Verification items for this drawing (mm, ordinates from the low corner). Coordinates: 2 decimals unless noted, no trailing zeros. Order: outer loops, then holes, each group sorted by start corner. A loop starts at its lowest first (then second) coordinate and runs counter-clockwise, first axis right, second up. Notation, with made-up numbers: M 36.5,-5.5 L 82.5,-5.5 A17 cw 82.5,19.5 Z; hole C 46,3 d11. An arc over 180 degrees is marked long. Use CSV: the item, a comma, the result in double quotes. Start each with the question number.
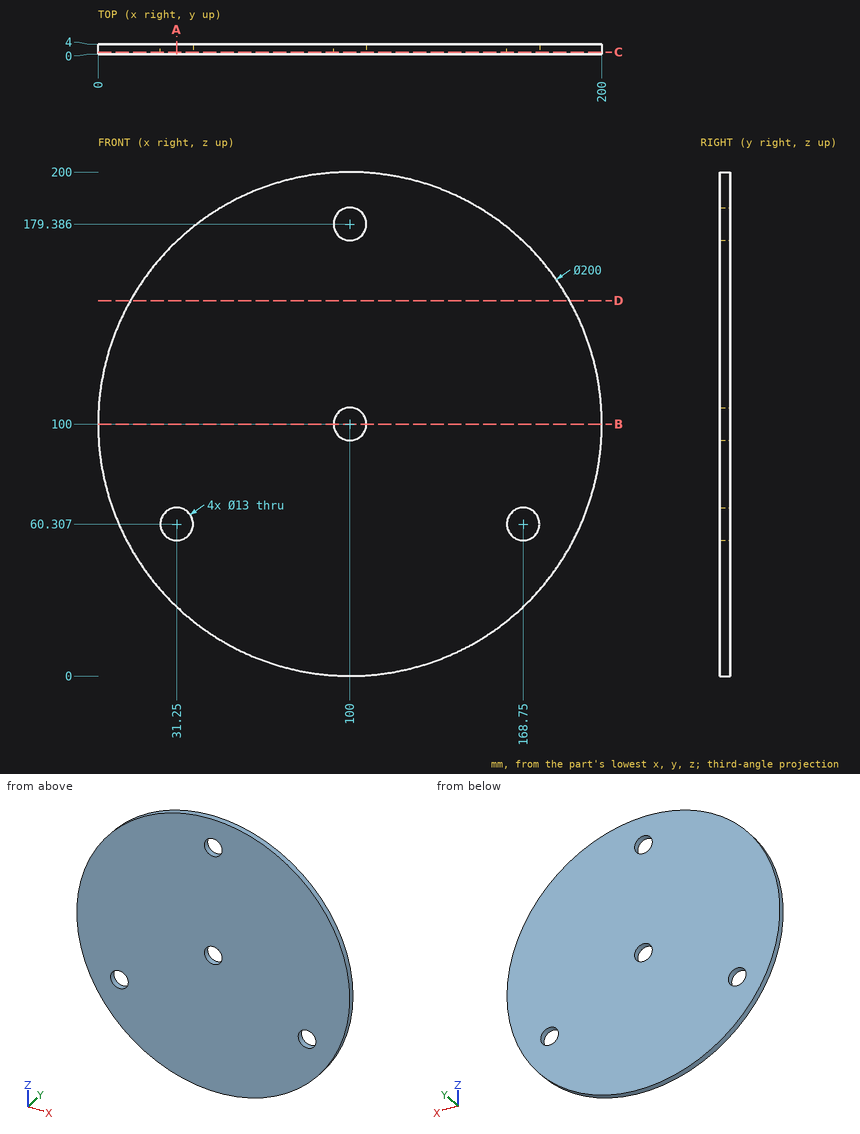
1) Section check B-B on z = 100. Record the boundary of the cut face in (x, y), then the cut area to 3 significant figures.
2) Section check D-D on z = 149. Record the boundary of the cut face in (x, y).
3) Material ranges on line 1 along Z through (x, y) = (100, 1.5) (1 decimal); line 2 along X through (y, z) = (0.2, 59); line 3 along Z through (x, y) = (31.25, 0.8), recorded low to high.
4) Section check C-C on y = 0.75. State how many separate pieces and enclosed holes the cut face has, then the cut area to 3 significant figures.
5) Section check A-A on x = 31.25. Record the boundary of the cut face in (y, z), then the cut area to 3 significant figures.
6) Gauge pin test, flat end, axial feed: P1, Ø1, axis at y = 3, z = 48.5, coming from the -X side. Record the tip position at first contact, or that the pin passes through.
Results are:
1,outline,"M 0,0 L 93.5,0 L 93.5,4 L 0,4 Z; M 106.5,0 L 200,0 L 200,4 L 106.5,4 Z"
1,area,"748 mm²"
2,outline,"M 12.83,0 L 187.17,0 L 187.17,4 L 12.83,4 Z"
3,line 1,"z = 0 to 93.5, 106.5 to 172.9, 185.9 to 200"
3,line 2,"x = 8.79 to 24.88, 37.62 to 162.38, 175.12 to 191.21"
3,line 3,"z = 27.38 to 53.81, 66.81 to 172.62"
4,separate pieces,"1"
4,enclosed holes,"4"
4,area,"30,900 mm²"
5,outline,"M 0,27.38 L 4,27.38 L 4,53.81 L 0,53.81 Z; M 0,66.81 L 4,66.81 L 4,172.62 L 0,172.62 Z"
5,area,"529 mm²"
6,P1,"stops at x = 13.98"
